Geometry check sheet. Reference: the model listing, model coordinates, mm. Face numbers are marked on the shaded views. A direction names the side the tool comes from. Coordinates: 2 decimals unless noted, no trailing zeros. Loops run counter-clockwise (first coordinate to the right, second up) from the corner with the lowest first, then second, coordinate; pieces in that order, holes last.
Autodesk Inventor part; units mm, degrees
ref_plane "YZ Plane" through (0, 0, 0) normal (1, 0, 0) x (0, 1, 0)
ref_plane "XZ Plane" through (0, 0, 0) normal (0, 1, 0) x (-1, 0, 0)
ref_plane "XY Plane" through (0, 0, 0) normal (0, 0, 1) x (1, 0, 0)
sketch "Sketch1" plane through (0, 0, 0) normal (0, 0, 1) x (1, 0, 0)
  line L0 (8.2804, 14.6939) -> (-8.2804, 14.6939)
  circle A0 centre (0, 0) radius 4.7752
  line L1 (-7.8994, -15.0749) -> (-5.3848, -15.0749)
  line L2 (-5.3848, -15.0749) -> (-5.3848, -22.3393)
  line L3 (8.2804, -15.4559) -> (5.7658, -15.4559)
  line L4 (5.7658, -15.4559) -> (5.7658, -22.3393)
  line L5 (5.7658, -22.3393) -> (-5.3848, -22.3393)
  arc A1 (-10.6934, -4.8641) -> (-11.0744, 4.0859) centre (-10.6934, -0.381) ccw
  line L6 (-11.0744, 11.8999) -> (-11.0744, 4.0859)
  line L7 (-10.6934, -4.8641) -> (-10.6934, -12.2809)
  arc A2 (11.0744, 4.1021) -> (11.0744, -4.8641) centre (11.0744, -0.381) ccw
  line L8 (11.0744, -12.6619) -> (11.0744, -4.8641)
  line L9 (11.0744, 4.1021) -> (11.0744, 11.8999)
  arc A3 (-8.2804, 14.6939) -> (-11.0744, 11.8999) centre (-8.2804, 11.8999) ccw
  arc A4 (11.0744, 11.8999) -> (8.2804, 14.6939) centre (8.2804, 11.8999) ccw
  arc A5 (8.2804, -15.4559) -> (11.0744, -12.6619) centre (8.2804, -12.6619) ccw
  arc A6 (-10.6934, -12.2809) -> (-7.8994, -15.0749) centre (-7.8994, -12.2809) ccw
  circle A7 centre (-8.2804, 11.8999) radius 1.3335
  circle A8 centre (8.2804, 11.8999) radius 1.3335
  circle A9 centre (8.2804, -12.6619) radius 1.3335
  circle A10 centre (-7.8994, -12.2809) radius 1.3335
  point P0 (-10.6934, -15.0749)
  point P1 (11.0744, 14.6939)
  point P2 (11.0744, -15.4559)
  point P3 (-11.0744, 14.6939)
  dimension "d0" = 30.1498
  dimension "d1" = 22.1488
  dimension "d2" = 9.5504
  dimension "d3" = 5.3086
  dimension "d4" = 7.2644
  dimension "d5" = 5.3086
  dimension "d6" = 8.9662
  dimension "d7" = 8.9662
  dimension "d11" = 2.794
  dimension "d12" = 2.667
  dimension "d13" = 2.667
  dimension "d14" = 2.667
  dimension "d15" = 2.667
extrude "Extrusion1" add sketch "Sketch1" along normal blind 2.54
fillet "Fillet1" radius 3.175 1 edges at (0.1905, -22.3393, 2.54)
sketch "Sketch2" plane through (0, 0, 0) normal (0, 0, -1) x (-1, 0, 0)
  line L0 (-5.7658, -19.2284) -> (5.3848, -19.2284)
  line L1 (-5.7658, -19.2284) -> (5.3848, -19.2284)
  line L2 (-5.7658, -22.3393) -> (-5.7658, -19.2284)
  line L3 (-5.7658, -19.2284) -> (-5.7658, -22.3393)
  line L4 (-5.7658, -22.3393) -> (5.3848, -22.3393)
  line L5 (-5.7658, -22.3393) -> (5.3848, -22.3393)
  line L6 (5.3848, -19.2284) -> (5.3848, -22.3393)
  line L7 (5.3848, -22.3393) -> (5.3848, -19.2284)
  point P0 (0, 0)
extrude "Extrusion2" add sketch "Sketch2" along normal blind 5.334
sketch "Sketch6" plane through (-5.3848, -22.3393, 0) normal (0, -1, 0) x (1, 0, 0)
  line L0 (11.1506, -5.334) -> (13.3604, -5.334)
  line L1 (16.1544, -8.128) -> (16.1544, -13.335)
  line L2 (0, -5.334) -> (-2.2098, -5.334)
  line L3 (-5.0038, -8.128) -> (-5.0038, -13.335)
  line L4 (-1.8288, -16.51) -> (12.9794, -16.51)
  line L5 (0, -5.334) -> (11.1506, -5.334)
  line L6 (0, -5.334) -> (11.1506, -5.334)
  arc A0 (12.9794, -16.51) -> (16.1544, -13.335) centre (12.9794, -13.335) ccw
  arc A1 (-5.0038, -13.335) -> (-1.8288, -16.51) centre (-1.8288, -13.335) ccw
  arc A2 (16.1544, -8.128) -> (13.3604, -5.334) centre (13.3604, -8.128) ccw
  arc A3 (-2.2098, -5.334) -> (-5.0038, -8.128) centre (-2.2098, -8.128) ccw
  point P0 (5.3848, 0)
  point P1 (16.1544, -5.334)
  point P2 (16.1544, -16.51)
  point P3 (-5.0038, -5.334)
  point P4 (-5.0038, -16.51)
  dimension "d30" = 5.0038
  dimension "d32" = 5.0038
  dimension "d35" = 3.175
  dimension "d36" = 2.794
extrude "Extrusion3" add sketch "Sketch6" against normal blind 3.1115
sketch "Sketch7" plane through (-5.3848, -19.2278, 0) normal (0, 1, 0) x (1, 0, 0)
  line L0 (0, 5.334) -> (11.1506, 5.334)
  line L1 (-1.8288, 16.51) -> (12.9794, 16.51)
  line L2 (3.9624, 12.9323) -> (3.9624, 3.1787)
  line L3 (7.1882, 3.1787) -> (7.1882, 12.9323)
  arc A0 (7.1882, 12.9323) -> (3.9624, 12.9323) centre (5.5753, 12.9323) ccw
  arc A1 (3.9624, 3.1787) -> (7.1882, 3.1787) centre (5.5753, 3.1787) ccw
  point P0 (5.3848, 0)
  point P1 (5.5753, 8.0555)
  dimension "d37" = 9.7536
  dimension "d38" = 3.2258
extrude "Extrusion4" cut sketch "Sketch7" against normal blind 76.2
sketch "Sketch8" plane through (-5.3848, -19.2278, 0) normal (0, 1, 0) x (1, 0, 0)
  circle A0 centre (13.3829, 13.3417) radius 1.4351
  circle A1 centre (13.3829, 8.1013) radius 1.4355
  circle A2 centre (-2.1844, 8.1013) radius 1.4351
  circle A3 centre (-2.1844, 13.3417) radius 1.4351
  point P0 (5.3848, 0)
  dimension "d48" = 2.8702
  dimension "d49" = 2.8702
  dimension "d50" = 2.8702
extrude "Extrusion5" cut sketch "Sketch8" against normal blind 76.2
properties part number "cwmotorholder"
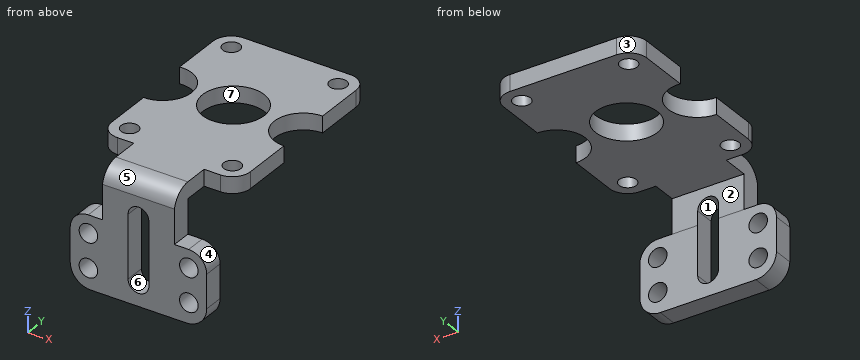
1) Section check B-B on y = 0. Record the cut outline in (x, z), and give its area (3 significant figures).
Data:
outline: (-6.23, 0) - (-4.78, 0) - (-4.78, 2.54) - (-6.23, 2.54) - close; (4.78, 0) - (6.61, 0) - (6.61, 2.54) - (4.78, 2.54) - close
area: 8.34 mm2
2) Section check A-A on z = -4. Record the cut outline in (x, y), and give its area (3 significant figures).
Data:
outline: (-5.38, -22.34) - (-1.42, -22.34) - (-1.42, -19.23) - (-5.38, -19.23) - close; (1.8, -22.34) - (5.77, -22.34) - (5.77, -19.23) - (1.8, -19.23) - close
area: 24.7 mm2
3) Section check D-D on z = 1.75. Record the cut outline in (x, y).
Data:
outline: (-11.07, 4.09) arc R4.48 cw (long way) to (-10.69, -4.86) - (-10.69, -12.28) arc R2.79 ccw to (-7.9, -15.07) - (-5.38, -15.07) - (-5.38, -21.32) - (5.77, -21.32) - (5.77, -15.46) - (8.28, -15.46) arc R2.79 ccw to (11.07, -12.66) - (11.07, -4.86) arc R4.48 cw to (11.07, 4.1) - (11.07, 11.9) arc R2.79 ccw to (8.28, 14.69) - (-8.28, 14.69) arc R2.79 ccw to (-11.07, 11.9) - close; hole circle Ø2.67 at (-8.28, 11.9); hole circle Ø2.67 at (-7.9, -12.28); hole circle Ø9.55 at (0, 0); hole circle Ø2.67 at (8.28, -12.66); hole circle Ø2.67 at (8.28, 11.9)
4) Material ranges on probe 1 along X at (y, z) = (12.5, 0.75); probe 2 along Z at (x, y) = (-4, -16.5); probe 3 along Y at (x, z) = (10, -10.5), recorded low to high.
Data:
probe 1: x = -11.01 to -9.47, -7.09 to 7.09, 9.47 to 11.01
probe 2: z = 0 to 2.54
probe 3: y = -22.34 to -19.23
5) Access from +Z, -Z, +X, -X, +Y, -Y to the whole of each face (thin tool, end or side, straight path). Record for the marked faces 1, 2 and 3.
Data:
face 1: +Y, -Y
face 2: -Z, +X, -X, +Y
face 3: +Z, -Z, -X, +Y
6) Mould release check, pull along X, two halves, no side actions. Record for the marked faces 4, 5, 6 and 7: +X half, -X half, draft (parallel to the pull), parting line (faces both ways), or undercut.
Data:
face 4: +X half
face 5: draft
face 6: undercut
face 7: undercut
7) Depth check by flat-ended pin: pin 1 (4 mm diameter, centred on x = 3, z = -7.5, fed in from +Y); pin 2 (2.5 mm diameter, centred on x = -3.5, y = -21.5, fed in from +Z); pin 3 (12.5 mm diameter, centred on x = 0, y = 0, fed in from +Z); pin 4 (3 mm diameter, centred on x = 8.28, y = -12.66, fed in from -Z). Enter the tip coordinate at first touch or a pass-through.
Data:
pin 1: stops at y = -19.23
pin 2: stops at z = 2.37
pin 3: stops at z = 2.54
pin 4: stops at z = 0
8) Section check C-C on x = -0.25. Record the cut outline in (y, z) (3 decimals).
Data:
outline: (-22.339, -16.51) - (-19.228, -16.51) - (-19.228, -14.484) - (-22.339, -14.484) - close; (-22.339, -1.627) - (-19.228, -1.627) - (-19.228, 0) - (-4.769, 0) - (-4.769, 2.54) - (-19.228, 2.54) arc R3.175 ccw to (-22.339, 0) - close; (4.769, 0) - (14.694, 0) - (14.694, 2.54) - (4.769, 2.54) - close
